Work out the finished part from the listing and answer in its coordinate system (mm). A direction names the side the tool comes from. Coordinates: 2 decimals unless noted, no trailing zeros. Order: outer loops, then holes, each group sorted by start corner. A loop starts at its lowest first (then second) coordinate and runs counter-clockwise, first axis right, second up. Notation, with made-up numbers: M 48,29 L 93,29 A21 ccw 93,59 Z; hole C -25.5,24.5 d11. An arc over 180 degrees is marked long. Use a Markdown table: item, result.
from build123d import *

# Parameters (mm, degrees)
BOSS_EXTRUDE1_DEPTH = 200
SHELL1_T            = -6
SKETCH4_W           = 600
SKETCH4_H           = 200
BOSS_EXTRUDE2_DEPTH = 2


with BuildPart() as part:
    # Sketch3 → Boss-Extrude1 (new body)
    with BuildSketch(Plane.XY):
        Polygon((9.153032832, -66.666666667), (329.933331479, -206.666666667), (609.153032832, -206.666666667), (609.153032832, 193.333333333), (9.153032832, 193.333333333), align=None)
    extrude(amount=BOSS_EXTRUDE1_DEPTH)

    # Shell1
    shell1_openings = [part.faces().sort_by_distance(p)[0] for p in [
        (309.153032832, 193.333333333, 100),
    ]]
    offset(amount=SHELL1_T, openings=shell1_openings, kind=Kind.INTERSECTION)

    # Sketch4 → Boss-Extrude2 (add)
    with BuildSketch(Plane(origin=(0, 193.333333333, 0), x_dir=(1, 0, 0), z_dir=(0, 1, 0))):
        with Locations((309.153032832, -100)):
            Rectangle(SKETCH4_W, SKETCH4_H)
    extrude(amount=BOSS_EXTRUDE2_DEPTH)


solid = part.part
1. Section A-A on x = 351 is taken. Determine the outline of the cut face in (y, z).
Answers below:
| item | result |
|---|---|
| outline | M -206.67,0 L 195.33,0 L 195.33,200 L -206.67,200 Z; hole M -200.67,6 L 193.33,6 L 193.33,194 L -200.67,194 Z |
2. For a pull along Z with two mould halves and no side action, classify faces 3 (the face through (305, -8, 0)), 4 (the face through (305, -1, 6)), 5 (the face through (167.298, -135.687, 98.6)) as +Z half, -Z half, draft (parallel to the pull), parting line (faces both ways), or undercut.
Answers below:
| item | result |
|---|---|
| face 3 | -Z half |
| face 4 | undercut |
| face 5 | draft |
3. For faces 1 (the face through (305, 195.333, 99)), 2 (the face through (305, 193.333, 99)), determine the directions among +Z, -Z, +X, -X, +Y, -Y from which every point of the face is accessible in a straight line to the end or side of a thin tool.
Answers below:
| item | result |
|---|---|
| face 1 | +Z, -Z, +X, -X, +Y |
| face 2 | none |
4. Section C-C on z = 53.5 is taken. Determine the outline of the cut face in (x, y), then the cut area to 3 significant figures.
Answers below:
| item | result |
|---|---|
| outline | M 9.15,-66.67 L 329.93,-206.67 L 609.15,-206.67 L 609.15,195.33 L 9.15,195.33 Z; hole M 15.15,-62.74 L 331.19,-200.67 L 603.15,-200.67 L 603.15,193.33 L 15.15,193.33 Z |
| area | 8,870 mm² |
5. Section B-B on y = 99 is taken. Determine the outline of the cut face in (x, z), then the cut area to 3 significant figures.
Answers below:
| item | result |
|---|---|
| outline | M 9.15,0 L 609.15,0 L 609.15,200 L 9.15,200 Z; hole M 15.15,6 L 603.15,6 L 603.15,194 L 15.15,194 Z |
| area | 9,460 mm² |
6. Find the intervals of material crossed by probe 1 along Z at (x, y) = (339.5, 108.5); probe 2 along X at (y, z) = (172, 109); probe 3 along Y at (x, z) = (353, 176.5), in increasing order.
Answers below:
| item | result |
|---|---|
| probe 1 | 0 to 6, 194 to 200 |
| probe 2 | 9.15 to 15.15, 603.15 to 609.15 |
| probe 3 | -206.67 to -200.67, 193.33 to 195.33 |
7. A flat-ended cylindrical pin translates along its axis: P1, Ø8, axis at x = 389, y = -65, coming from the -Z side. Find the tip coordinate at first contact, or state that the pin passes through.
Answers below:
| item | result |
|---|---|
| P1 | z = 0 |
